The drawing under review shows one solid part. Ordinate dimensions are in mm from its lowest x, y, z. Round coordinates to 2 decimals unless told otherwise and drop trailing zeros. Order: outer loops, then holes, each group sorted by start corner. A loop starts at its lowest first (then second) coordinate and runs counter-clockwise, first axis right, second up.
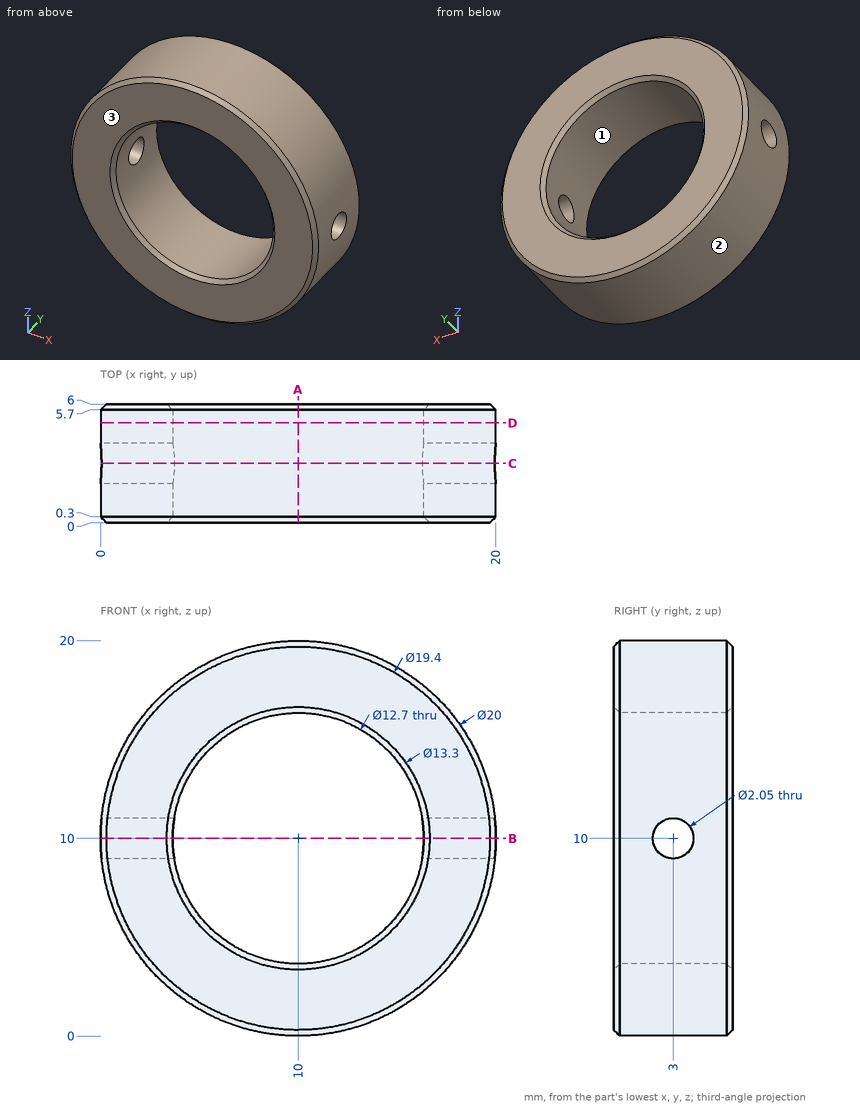
(1) We need section A-A (x = 10). Give the boundary of the cut face in (y, z), and give its area (3 significant figures).
(2) We need section D-D (y = 5.05). Give the boundary of the cut face in (x, z), and give its area (3 significant figures).
(3) We need section C-C (y = 3). Give the boundary of the cut face in (x, z) (3 decimals).
(4) To check wall thickness, follow L1, parallel to X at y = 5.1, z = 10.25; L2, parallel to Z at x = 2.4, y = 3 (3 decimals); L3, parallel to Z at x = 9, y = 4.3. State the ranges of each line that lie inside material, in increasing order.
(5) Clearance check with flat-ended pins moving along their axes: P1, Ø1.8, axis at y = 3, z = 10, coming from the -X side; P2, Ø3, axis at y = 2, z = 4, coming from the +X side; P3, Ø1, axis at x = 9, y = 5, coming from the +Z side; P4, Ø12, axis at x = 7, z = 16, coming from the -Y side. State where each tip first meets the part, or that it passes through.
(6) We need section B-B (z = 10). Give the boundary of the cut face in (x, y) (3 decimals), and give its area (3 significant figures).
(7) The part is to be moulded in two halves that separate along X. For the marked faces 1, 2 and 3, say which applies: pulls with the +X half, pulls with the -X half, needs draft (parallel to the pull), parting line crosses it, or undercut.
Verdict:
1. outline: (0, 0.3) - (0.3, 0) - (5.7, 0) - (6, 0.3) - (6, 3.35) - (5.7, 3.65) - (0.3, 3.65) - (0, 3.35) - close; (0, 16.65) - (0.3, 16.35) - (5.7, 16.35) - (6, 16.65) - (6, 19.7) - (5.7, 20) - (0.3, 20) - (0, 19.7) - close
1. area: 43.4 mm2
2. outline: circle Ø20 at (10, 10); hole circle Ø12.7 at (10, 10)
2. area: 187 mm2
3. outline: (0.053, 8.975) arc R10 ccw to (19.947, 8.975) - (16.267, 8.975) arc R6.35 cw to (3.733, 8.975) - close; (0.053, 11.025) - (3.733, 11.025) arc R6.35 cw to (16.267, 11.025) - (19.947, 11.025) arc R10 ccw to start
4. L1: x = 0 to 3.65, 16.35 to 20
4. L2: z = 3.501 to 8.975, 11.025 to 16.499
4. L3: z = 0.05 to 3.73, 16.27 to 19.95
5. P1: passes through
5. P2: stops at x = 18.93
5. P3: stops at z = 19.99
5. P4: stops at y = 0
6. outline: (0, 0.3) - (0.3, 0) - (3.35, 0) - (3.65, 0.3) - (3.65, 1.975) - (0, 1.975) - close; (0, 4.025) - (3.65, 4.025) - (3.65, 5.7) - (3.35, 6) - (0.3, 6) - (0, 5.7) - close; (16.35, 0.3) - (16.65, 0) - (19.7, 0) - (20, 0.3) - (20, 1.975) - (16.35, 1.975) - close; (16.35, 4.025) - (20, 4.025) - (20, 5.7) - (19.7, 6) - (16.65, 6) - (16.35, 5.7) - close
6. area: 28.5 mm2
7. face 1: undercut
7. face 2: parting line crosses it
7. face 3: needs draft
